Answer from the drawing. Dimensions are ordinates in mm from the lowest x, y and z of the part. A direction names the side the tool comes from. Give positions to 0.01 mm unless a question says otherwise; leave off trailing zeros. Order: outer loops, then holes, each group sorted by start corner. A loop starts at its lowest first (then second) coordinate and runs counter-clockwise, first axis right, second up. Notation, with made-up numbers: (61.25, -25) -> (93.25, -25) arc R25 cw to (93.25, 13) -> close; hole circle Ø1 at (6, 72). An arc over 180 degrees is marked (long way). Answer as CSV lines item,"result". Start each with the question number.
1) Find section D-D (z = 12). Determine the outline of the cut face in (x, y).
2) Find section C-C (x = 9.75). Determine the outline of the cut face in (y, z) (1 decimal).
3) Flat-ended cylindrical pins translate along their axes: pin 1 Ø5 at (x, y) = (9.5, 12) entering from +Z; pin 2 Ø1 at (x, y) = (6.5, 9.5) entering from -Z; pin 3 Ø2 at (x, y) = (10.5, 9) entering from +Z (1 decimal). Find the tip coordinate at first contact, or state that the pin passes through.
4) Find section B-B (z = 6.75). Determine the outline of the cut face in (x, y) (1 decimal), and give its area (3 significant figures).
5) Straight lines are drawn through the part: L1, parallel to Y at x = 13, z = 13; L2, parallel to Z at x = 10.25, y = 3.5 (1 decimal); L3, parallel to X at y = 14.5, z = 7.5. For each, find the intervals that lie inside material, in ascending order. Write a range as from..to.
6) Find section A-A (y = 1). Determine the outline of the cut face in (x, z) (1 decimal).
7) For the marked faces 1 and 2, determine the directions among +Z, -Z, +X, -X, +Y, -Y from which every point of the face is accessible in a straight line to the end or side of a thin tool.
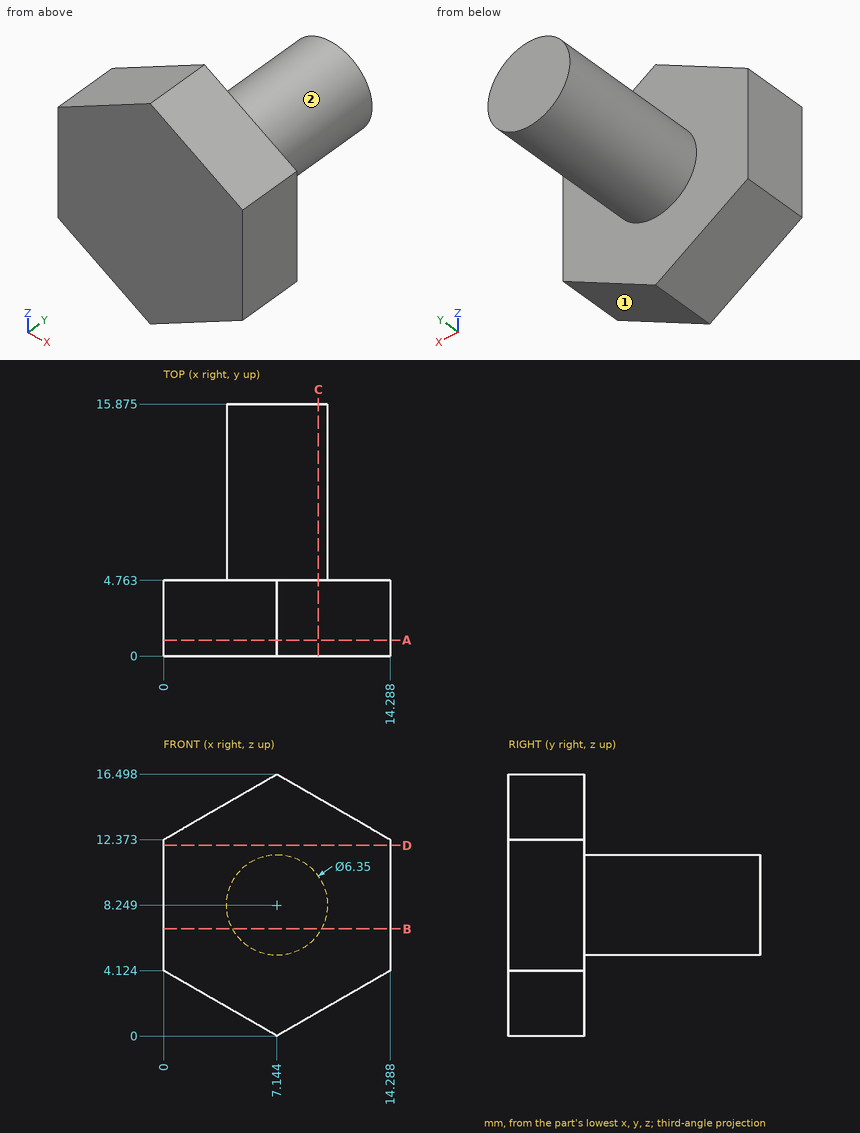
Findings below:
1,outline,"(0, 0) -> (14.29, 0) -> (14.29, 4.76) -> (0, 4.76) -> close"
2,outline,"(0, 1.5) -> (4.8, 1.5) -> (4.8, 6.4) -> (15.9, 6.4) -> (15.9, 10.1) -> (4.8, 10.1) -> (4.8, 15) -> (0, 15) -> close"
3,pin 1,"z = 11.42"
3,pin 2,"z = 5.08"
3,pin 3,"z = 10.4"
4,outline,"(0, 0) -> (14.3, 0) -> (14.3, 4.8) -> (9.9, 4.8) -> (9.9, 15.9) -> (4.3, 15.9) -> (4.3, 4.8) -> (0, 4.8) -> close"
4,area,"130 mm²"
5,L1,"0..4.76"
5,L2,"1.8..14.7"
5,L3,"4.06..10.23"
6,outline,"(0, 4.1) -> (7.1, 0) -> (14.3, 4.1) -> (14.3, 12.4) -> (7.1, 16.5) -> (0, 12.4) -> close"
7,face 1,"-Z, +X, +Y, -Y"
7,face 2,"+Y"
